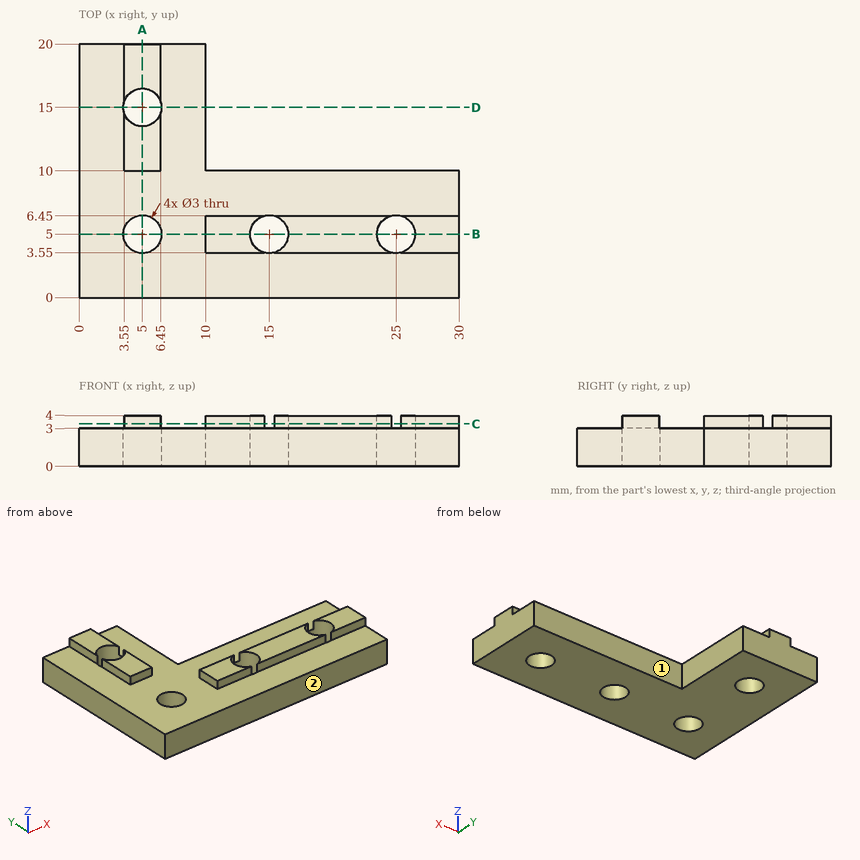
Check sheet for the drawn part. Datum: minimum x, y, z corner. Units: mm. A direction names the side the tool comes from. Round coordinates to 2 decimals unless told otherwise and drop trailing zeros. Order: outer loops, then holes, each group sorted by start corner. A loop starts at its lowest first (then second) coordinate and runs counter-clockwise, first axis right, second up. Notation, with made-up numbers: M 43.25,54.25 L 88.25,54.25 A19 ccw 88.25,71.25 Z; hole C -28,-33 d8. An arc over 180 degrees is marked long. Write each question's results on one line, items separated by ' | '. Start each with the question number.
1. Go/stop test with flat-tipped pins: P1, Ø0.5, axis at y = 17.5, z = 3.5, coming from the -X side; P2, Ø1.8, axis at x = 25, y = 5, coming from the -Z side; P3, Ø0.8, axis at y = 13, z = 3.5, coming from the +X side; P4, Ø1.1, axis at x = 20, z = 3.5, coming from the +Y side. Record where each tip stops, or that it passes through.
2. Cross-section at D-D on y = 15. Record the boundary of the cut face in (x, z).
3. Material ranges on L1, parallel to Y at x = 5, z = 0.8; L2, parallel to Y at x = 25, z = 2.95, recorded low to high. Write a range as from..to.
4. Set-up check for the marked faces 1 and 2: record each of +Z, -Z, +X, -X, +Y, -Y from which the full face is reachable in a straight line by a thin tool's end or side.
5. Cross-section at B-B on y = 5. Record the boundary of the cut face in (x, z), plus the area to 3 significant figures.
6. Cross-section at C-C on z = 3.35. Record the boundary of the cut face in (x, y), plus the area to 3 significant figures.
7. Cross-section at A-A on x = 5. Record the boundary of the cut face in (y, z).
Resolved:
1) P1: x = 3.55 | P2: through | P3: x = 6.45 | P4: y = 10
2) outline: M 0,0 L 3.5,0 L 3.5,3 L 0,3 Z; M 6.5,0 L 10,0 L 10,3 L 6.5,3 Z
3) L1: 0..3.5, 6.5..13.5, 16.5..20 | L2: 0..3.5, 6.5..10
4) face 1: +Z, -Z, +X, +Y | face 2: +Z, -Z, +X, -X, -Y
5) outline: M 0,0 L 3.5,0 L 3.5,3 L 0,3 Z; M 6.5,0 L 13.5,0 L 13.5,4 L 10,4 L 10,3 L 6.5,3 Z; M 16.5,0 L 23.5,0 L 23.5,4 L 16.5,4 Z; M 26.5,0 L 30,0 L 30,4 L 26.5,4 Z | area: 77.0 mm2
6) outline: M 3.55,10 L 6.45,10 L 6.45,14.62 A1.5 cw 3.55,14.62 Z; M 3.55,15.38 A1.5 cw 6.45,15.38 L 6.45,20 L 3.55,20 Z; M 10,3.55 L 14.62,3.55 A1.5 cw 14.62,6.45 L 10,6.45 Z; M 15.38,3.55 L 24.62,3.55 A1.5 cw 24.62,6.45 L 15.38,6.45 A1.5 cw Z; M 25.38,3.55 L 30,3.55 L 30,6.45 L 25.38,6.45 A1.5 cw Z | area: 65.9 mm2
7) outline: M 0,0 L 3.5,0 L 3.5,3 L 0,3 Z; M 6.5,0 L 13.5,0 L 13.5,4 L 10,4 L 10,3 L 6.5,3 Z; M 16.5,0 L 20,0 L 20,4 L 16.5,4 Z
